Input: part model. Units: mm. Frame: model coordinates. A direction names the side the tool comes from. Give positions to 0.01 mm unless a question says otherwise; leave off trailing zeros. Loops run counter-clockwise (first coordinate to the right, second up) from the corner with the lowest first, then second, coordinate; pieces in that order, holes last. Notation, with made-up numbers: M -36,15 L -15,15 A27 cw -15,38 Z; hole C 28,-27 d2. An arc over 180 degrees is marked long. Answer as a JSON object with one key per item and string values. Group by question number.
```python
from build123d import *

# Parameters (mm, degrees)
BOSS_EXTRUDE1_DEPTH = 2.54
CUT_EXTRUDE1_START  = 2.54
SKETCH5_W           = 228.6
SKETCH5_H           = 3.175
CUT_EXTRUDE1_DEPTH  = 2.54
SKETCH6_W           = 248.92
SKETCH6_H           = 1.905
BOSS_EXTRUDE3_DEPTH = 12.7


with BuildPart() as part:
    # Sketch3 → Boss-Extrude1 (new body)
    with BuildSketch(Plane(origin=(0, 0, 0), x_dir=(1, 0, 0), z_dir=(0, 1, 0))):
        with BuildLine():
            Line((-124.46, 19.05), (124.46, 19.05))
            ThreePointArc((124.46, 19.05), (126.256051224, 18.306051224), (127, 16.51))
            Line((127, 16.51), (127, -16.51))
            ThreePointArc((127, -16.51), (126.256051224, -18.306051224), (124.46, -19.05))
            Line((124.46, -19.05), (-124.46, -19.05))
            ThreePointArc((-124.46, -19.05), (-126.256051224, -18.306051224), (-127, -16.51))
            Line((-127, -16.51), (-127, 16.51))
            ThreePointArc((-127, 16.51), (-126.256051224, 18.306051224), (-124.46, 19.05))
        make_face()
    extrude(amount=BOSS_EXTRUDE1_DEPTH)

    # Sketch5 → Cut-Extrude1 (cut)
    with BuildSketch(Plane(origin=(0, 0, 0), x_dir=(1, 0, 0), z_dir=(0, 1, 0)).offset(CUT_EXTRUDE1_START)):
        Rectangle(SKETCH5_W, SKETCH5_H)
    extrude(amount=-CUT_EXTRUDE1_DEPTH, mode=Mode.SUBTRACT)

    # Sketch6 → Boss-Extrude3 (add)
    with BuildSketch(Plane.XZ):
        with Locations((0, -2.54)):
            Rectangle(SKETCH6_W, SKETCH6_H)
        with Locations((0, 2.54)):
            Rectangle(SKETCH6_W, SKETCH6_H)
    extrude(amount=BOSS_EXTRUDE3_DEPTH)


solid = part.part
```
1. Section C-C (z = 7.5). Output: boundary loops of the cut face in (x, y).
2. First-contact query: P1, Ø1.5, axis at x = -21, y = -10, coming from the -Z side; P2, Ø2, axis at x = -95.5, z = 11, coming from the -Y side; P3, Ø4, axis at x = -33.5, y = -8.5, coming from the +Z side; P4, Ø4, axis at y = -4.5, z = 7, coming from the +X side. Flat tips, straight axial feed; report the tip coordinate or a pass-through.
3. Reachability of faces 3 (the flat face through (-2, -6, 3.492)), 4 (the flat face through (2, 2.54, -5)) from +Z, -Z, +X, -X, +Y, -Y: full face, straight path, thin tool, end or side. Return the list, or none.
4. Section B-B (x = 87.5). Output: boundary loops of the cut face in (y, z), then the cut area to 3 significant figures.
5. Mould query, pull axis X, two halves, no side actions, for faces 1 (the flat face through (-2, -6, -3.492)), 2 (the flat face through (-2, -5, 1.588)). Classes: pulls with the +X half, pulls with the -X half, needs draft (parallel to the pull), parting line crosses it, or undercut.
6. Material intervals for L1, parallel to Z at x = 18.5, y = -1.5; L2, parallel to Z at x = -74.5, y = 0.25; L3, parallel to Y at x = -55, z = 15, sorted ascending.
7. Section A-A (y = -6.5). Output: boundary loops of the cut face in (x, z).
Geometry results:
{
 "1": {"outline": "M -127,0 L 127,0 L 127,2.54 L -127,2.54 Z"},
 "2": {"P1": "z = -3.49", "P2": "y = 0", "P3": "z = 3.49", "P4": "through"},
 "3": {"face 3": "+Z, +X, -X, -Y", "face 4": "+Z, -Z, +X, -X, +Y"},
 "4": {"outline": "M -12.7,-3.49 L 0,-3.49 L 0,-19.05 L 2.54,-19.05 L 2.54,-1.59 L -12.7,-1.59 Z; M -12.7,1.59 L 2.54,1.59 L 2.54,19.05 L 0,19.05 L 0,3.49 L -12.7,3.49 Z", "area": "137 mm2"},
 "5": {"face 1": "needs draft", "face 2": "undercut"},
 "6": {"L1": "-3.49 to -1.59, 1.59 to 3.49", "L2": "-19.05 to -1.59, 1.59 to 19.05", "L3": "0 to 2.54"},
 "7": {"outline": "M -124.46,-3.49 L 124.46,-3.49 L 124.46,-1.59 L -124.46,-1.59 Z; M -124.46,1.59 L 124.46,1.59 L 124.46,3.49 L -124.46,3.49 Z"}
}
